```python
from build123d import *

# Parameters (mm, degrees)
SKETCH_1_W          = 72
SKETCH_1_H          = 50
EXTRUDE_1_DEPTH     = 25
SKETCH_3_R          = 1.5
CUT_EXTRUDE_1_DEPTH = 51.457903246
SKETCH_4_W          = 6
SKETCH_4_H          = 6
CUT_EXTRUDE_2_DEPTH = 20


with BuildPart() as part:
    # 草图1 → 凸台-拉伸1 (new body)
    with BuildSketch(Plane(origin=(0, 0, 0), x_dir=(1, 0, 0), z_dir=(0, 1, 0))):
        Rectangle(SKETCH_1_W, SKETCH_1_H)
    extrude(amount=EXTRUDE_1_DEPTH)

    # 草图3 → 切除-拉伸1 (cut, through all)
    with BuildSketch(Plane(origin=(0, 25, 0), x_dir=(1, 0, 0), z_dir=(0, 1, 0))):
        with Locations(Location((-33, 22, 0), (0, 0, 270))):
            Circle(SKETCH_3_R)
        with Locations(Location((33, 22, 0), (0, 0, 90))):
            Circle(SKETCH_3_R)
        with Locations(Location((33, -22, 0), (0, 0, 270))):
            Circle(SKETCH_3_R)
        with Locations(Location((-33, -22, 0), (0, 0, 90))):
            Circle(SKETCH_3_R)
    extrude(amount=-CUT_EXTRUDE_1_DEPTH, mode=Mode.SUBTRACT)

    # 草图4 → 切除-拉伸2 (cut)
    with BuildSketch(Plane(origin=(0, 25, 0), x_dir=(1, 0, 0), z_dir=(0, 1, 0))):
        with Locations((-33, 22)):
            Rectangle(SKETCH_4_W, SKETCH_4_H)
        with Locations((33, 22)):
            Rectangle(SKETCH_4_W, SKETCH_4_H)
        with Locations((33, -22)):
            Rectangle(SKETCH_4_W, SKETCH_4_H)
        with Locations((-33, -22)):
            Rectangle(SKETCH_4_W, SKETCH_4_H)
    extrude(amount=-CUT_EXTRUDE_2_DEPTH, mode=Mode.SUBTRACT)


solid = part.part
```
Geometry check sheet. Reference: the model listing, model coordinates, mm. A direction names the side the tool comes from. Coordinates: 2 decimals unless noted, no trailing zeros. Write each loop counter-clockwise with the first axis right and the second up, starting at its lowest first coordinate (ties: lowest second). Pieces come first, ordered by that corner, then holes. Notation, with made-up numbers: M -17.75,34 L 6.25,34 A29 ccw 6.25,71 Z; hole C 79.25,74.25 d10. An arc over 180 degrees is marked long. Use one line per item in the form item = value. Start each with the question number.
1) Thickness scan on probe 1 along X at (y, z) = (2.6, 22); probe 2 along Z at (x, y) = (-32.5, 12). Record the ranges inside material, lowest first. Write a range as from..to.
2) Set-up check for faces 1 (the flat face through (30, 15, 22)), 2 (the flat face through (-34.4, 5, 20.6)), 3 (the flat face through (-34.4, 5, -23.4)): record each of +Z, -Z, +X, -X, +Y, -Y from which the full face is reachable in a straight line by a thin tool's end or side.
3) Section check B-B on y = 21. Enter the section's corners in (x, z), and give its area (3 significant figures).
4) Go/stop test with flat-tipped pins: pin 1 Ø3 at (x, z) = (-32, 21.5) entering from +Y; pin 2 Ø4 at (x, z) = (-10.5, 2.5) entering from -Y; pin 3 Ø1.8 at (x, y) = (-34.5, 19.5) entering from -Z; pin 4 Ø1.8 at (y, z) = (13.5, 23.5) entering from +X. Record where each tip stops, or that it passes through.
5) Section check A-A on z = -22. Enter the section's corners in (x, y).
Responses:
q1.probe_1 = -36..-34.5, -31.5..31.5, 34.5..36
q1.probe_2 = -19..19
q2.face_1 = +Z, +X, +Y
q2.face_2 = +Z, -X, +Y
q2.face_3 = -Z, -X, +Y
q3.outline = M -36,-19 L -30,-19 L -30,-25 L 30,-25 L 30,-19 L 36,-19 L 36,19 L 30,19 L 30,25 L -30,25 L -30,19 L -36,19 Z
q3.area = 3,460 mm2
q4.pin_1 = 5
q4.pin_2 = 0
q4.pin_3 = -19
q4.pin_4 = 30
q5.outline = M -36,0 L -34.5,0 L -34.5,5 L -36,5 Z; M -31.5,0 L 31.5,0 L 31.5,5 L 30,5 L 30,25 L -30,25 L -30,5 L -31.5,5 Z; M 34.5,0 L 36,0 L 36,5 L 34.5,5 Z
